from build123d import *

# Parameters (mm, degrees)
F0_W          = 104
F0_H          = 84
F1_DEPTH      = 13
F3_R          = 9
F4_DEPTH      = 8
F5_R          = 4.5
F6_DEPTH      = 25
F7_R          = 27
F8_DEPTH      = 25
F9_R          = 13
F10_T1_DEPTH  = 58
F10_T3_DEPTH  = 78
F10_T6_ANGLE  = 90
F10_T8_ANGLE  = 90
F10_T10_ANGLE = 90
F10_T12_ANGLE = 90


# Not quite as in the source:
# - a fillet or chamfer that OpenCascade refuses, or shapes differently, is made with other operations: its cross-section is extruded or revolved along the edge and cut away or added


with BuildPart() as f1:
    # F0 (on Top) → F1 (new body)
    with BuildSketch(Plane.XY):
        Rectangle(F0_W, F0_H)
    extrude(amount=-F1_DEPTH)

    # F3 (on Top) → F4 (cut)
    with BuildSketch(Plane.XY):
        with Locations((38.3695703445, 28.125)):
            Circle(F3_R)
        with Locations((38.3695703445, -28.125)):
            Circle(F3_R)
        with Locations((-38.3695703445, 28.125)):
            Circle(F3_R)
        with Locations((-38.3695703445, -28.125)):
            Circle(F3_R)
    extrude(amount=-F4_DEPTH, mode=Mode.SUBTRACT)

    # F5 (on face) → F6 (cut)
    with BuildSketch(Plane.XY.offset(-8)):
        with Locations((38.3695703445, 28.125)):
            Circle(F5_R)
        with Locations((38.3695703445, -28.125)):
            Circle(F5_R)
        with Locations((-38.3695703445, 28.125)):
            Circle(F5_R)
        with Locations((-38.3695703445, -28.125)):
            Circle(F5_R)
    extrude(amount=-F6_DEPTH, mode=Mode.SUBTRACT)

    # F7 (on Top) → F8 (cut)
    with BuildSketch(Plane.XY):
        Circle(F7_R)
    extrude(amount=-F8_DEPTH, mode=Mode.SUBTRACT)

    # F9
    f9_edges = [f1.edges().sort_by_distance(p)[0] for p in [
        (-52, 42, -6.5),
        (-52, -42, -6.5),
        (52, -42, -6.5),
        (52, 42, -6.5),
    ]]
    fillet(f9_edges, radius=F9_R)

    # F10: fillet of radius 5 on 8 edges, made by hand

    # F10_s2 → F10_t1 (cut)
    with BuildSketch(Plane.XZ.offset(-29)):
        with BuildLine():
            ThreePointArc((-47, 0), (-50.5355339059, -1.4644660941), (-52, -5))
            Line((-52, -5), (-52, 0))
            Line((-52, 0), (-47, 0))
        make_face()
        with BuildLine():
            ThreePointArc((52, -5), (50.5355339059, -1.4644660941), (47, 0))
            Line((47, 0), (52, 0))
            Line((52, 0), (52, -5))
        make_face()
    extrude(amount=F10_T1_DEPTH, mode=Mode.SUBTRACT)

    # F10_s4 → F10_t3 (cut)
    with BuildSketch(Plane.YZ.offset(-39)):
        with BuildLine():
            ThreePointArc((-37, 0), (-40.5355339059, -1.4644660941), (-42, -5))
            Line((-42, -5), (-42, 0))
            Line((-42, 0), (-37, 0))
        make_face()
        with BuildLine():
            ThreePointArc((37, 0), (40.5355339059, -1.4644660941), (42, -5))
            Line((42, -5), (42, 0))
            Line((42, 0), (37, 0))
        make_face()
    extrude(amount=F10_T3_DEPTH, mode=Mode.SUBTRACT)

    # F10_s5 → F10_t6 (revolve, cut)
    with BuildSketch(Plane.XZ.offset(29)):
        with BuildLine():
            ThreePointArc((47, 0), (50.5355339059, -1.4644660941), (52, -5))
            Line((52, -5), (52, 0))
            Line((52, 0), (47, 0))
        make_face()
    revolve(axis=Axis((39, -29, 0), (0, 0, -1)), revolution_arc=F10_T6_ANGLE, mode=Mode.SUBTRACT)

    # F10_s7 → F10_t8 (revolve, cut)
    with BuildSketch(Plane.XZ.offset(-29)):
        with BuildLine():
            ThreePointArc((47, 0), (50.5355339059, -1.4644660941), (52, -5))
            Line((52, -5), (52, 0))
            Line((52, 0), (47, 0))
        make_face()
    revolve(axis=Axis((39, 29, 0), (0, 0, 1)), revolution_arc=F10_T8_ANGLE, mode=Mode.SUBTRACT)

    # F10_s9 → F10_t10 (revolve, cut)
    with BuildSketch(Plane.YZ.offset(-39)):
        with BuildLine():
            ThreePointArc((-37, 0), (-40.5355339059, -1.4644660941), (-42, -5))
            Line((-42, -5), (-42, 0))
            Line((-42, 0), (-37, 0))
        make_face()
    revolve(axis=Axis((-39, -29, 0), (0, 0, -1)), revolution_arc=F10_T10_ANGLE, mode=Mode.SUBTRACT)

    # F10_s11 → F10_t12 (revolve, cut)
    with BuildSketch(Plane.YZ.offset(-39)):
        with BuildLine():
            ThreePointArc((37, 0), (40.5355339059, -1.4644660941), (42, -5))
            Line((42, -5), (42, 0))
            Line((42, 0), (37, 0))
        make_face()
    revolve(axis=Axis((-39, 29, 0), (0, 0, 1)), revolution_arc=F10_T12_ANGLE, mode=Mode.SUBTRACT)


solid = f1.part
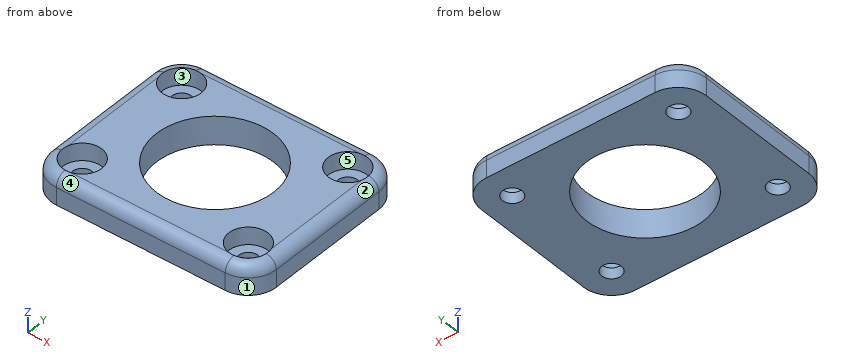
Could you check a few things on this model? Use its own coordinates, in mm. Face numbers are marked on the shaded views. A direction names the side the tool comes from. Give positions to 0.01 mm unless a question says otherwise; leave off trailing zeros. Order: outer loops, then holes, each group sorted by start corner. A loop starts at its lowest first (then second) coordinate and runs counter-clockwise, first axis right, second up. Notation, with made-up numbers: (60, 41) - (74, 41) arc R11 ccw to (74, 62) - close; hole circle Ø6 at (53, 49). An arc over 180 degrees is marked (long way). One line per question, with ' | ' between items. Start each with the question number.
Item 1: I want a section at C-C on z = -3.25. Write out the boundary of the cut face in (x, y) (1 decimal), then the cut area to 3 significant figures.
Item 2: I want a section at D-D on z = -11. Write out the boundary of the cut face in (x, y) (3 decimals), then the cut area to 3 significant figures.
Item 3: I need wall thicknesses on probe 1 along X at (y, z) = (1, -7); probe 2 along Y at (x, z) = (0, -7); probe 3 along X at (y, z) = (-21, -1). Which ranges of each line are inside material? Lowest first, please. Write a range as [from, to].
Item 4: For the marked faces 4 and 5, which set-ups out of +Z, -Z, +X, -X, +Y, -Y let a thin tool reach every point of the face, with its end or its side?
Item 5: I want a section at B-B on x = 0. Write out the boundary of the cut face in (y, z).
Item 6: I'm going to push flat-ended pins straight in: pin 1 Ø2 at (x, y) = (36.5, 3) entering from +Z; pin 2 Ø14.5 at (x, y) = (-38.37, -28.12) entering from +Z; pin 3 Ø3 at (y, z) = (-32.5, -6) entering from -X. Where does each tip first touch, or does it pass through?
Item 7: Thinking about a two-plate mould opening in Y: for the marked faces 1, 2 and 3, which applies, pulls with the +Y half, pulls with the -Y half, needs draft (parallel to the pull), parting line crosses it, or undercut?
Item 8: I want a section at A-A on y = 0. Write out the boundary of the cut face in (x, z).
Verdict:
1) outline: (-51.7, -29) arc R12.7 ccw to (-39, -41.7) - (39, -41.7) arc R12.7 ccw to (51.7, -29) - (51.7, 29) arc R12.7 ccw to (39, 41.7) - (-39, 41.7) arc R12.7 ccw to (-51.7, 29) - close; hole circle Ø18 at (-38.4, -28.1); hole circle Ø18 at (-38.4, 28.1); hole circle Ø54 at (0, 0); hole circle Ø18 at (38.4, -28.1); hole circle Ø18 at (38.4, 28.1) | area: 5,170 mm^2
2) outline: (-52, -29) arc R13 ccw to (-39, -42) - (39, -42) arc R13 ccw to (52, -29) - (52, 29) arc R13 ccw to (39, 42) - (-39, 42) arc R13 ccw to (-52, 29) - close; hole circle Ø9 at (-38.37, -28.125); hole circle Ø9 at (-38.37, 28.125); hole circle Ø54 at (0, 0); hole circle Ø9 at (38.37, -28.125); hole circle Ø9 at (38.37, 28.125) | area: 6,050 mm^2
3) probe 1: [-52, -26.98], [26.98, 52] | probe 2: [-42, -27], [27, 42] | probe 3: [-50, -43.87], [-32.87, -16.97], [16.97, 32.87], [43.87, 50]
4) face 4: +Z, +X, -X, -Y | face 5: +Z
5) outline: (-42, -13) - (-27, -13) - (-27, 0) - (-37, 0) arc R5 ccw to (-42, -5) - close; (27, -13) - (42, -13) - (42, -5) arc R5 ccw to (37, 0) - (27, 0) - close
6) pin 1: z = 0 | pin 2: z = -8 | pin 3: x = -51.85
7) face 1: pulls with the -Y half | face 2: needs draft | face 3: undercut
8) outline: (-52, -13) - (-27, -13) - (-27, 0) - (-47, 0) arc R5 ccw to (-52, -5) - close; (27, -13) - (52, -13) - (52, -5) arc R5 ccw to (47, 0) - (27, 0) - close
